```python
from build123d import *

# Parameters (mm, degrees)
F1_DEPTH = 25.4
F3_D     = 12.7
F5_D     = 12.7


with BuildPart() as f1:
    # F0 (on Front) → F1 (new body)
    with BuildSketch(Plane.XZ):
        Polygon((-34.180485, 31.123895), (-71.779169, 31.123895), (-71.779169, -31.123895), (71.779169, -31.123895), (71.779169, 31.123895), (29.286098, 31.123895), (29.286098, 4.353631), (-34.180485, 4.353631), align=None)
    extrude(amount=F1_DEPTH)

    # F3 (through all)
    with Locations(Plane.XY.offset(4.353631)):
        with Locations((0, -12.7)):
            Hole(F3_D / 2)

    # F5 (through all)
    with Locations(Plane(origin=(-71.779169, 0, 0), x_dir=(0, -1, 0), z_dir=(-1, 0, 0))):
        with Locations((12.7, 0)):
            Hole(F5_D / 2)


solid = f1.part
```
Geometry: final body of the model. Coordinates: model frame, mm. A direction names the side the tool comes from. Give positions to 0.01 mm unless a question says otherwise; leave off trailing zeros. Order: outer loops, then holes, each group sorted by start corner. A loop starts at its lowest first (then second) coordinate and runs counter-clockwise, first axis right, second up. Notation, with made-up numbers: (77.5, 89) -> (120.5, 89) arc R19 ccw to (120.5, 108) -> close; hole circle Ø11 at (-30.5, 77). An arc over 180 degrees is marked (long way). Write each question's results on one line, items separated by ' | '. Start each with the question number.
1) Draft query along Y for faces 1 (the flat face through (-1, -25.4, -6)), 2 (the flat face through (-1, 0, -6)), 3 (the cylindrical face through (-43.36, -14.08, -6.2)), 4 (the cylindrical face through (-0.07, -6.35, 2.63)). Return one class per face: pulls with the +Y half, pulls with the -Y half, needs draft (parallel to the pull), parting line crosses it, or undercut.
2) Line query: line 1 (X direction, y = -12.7, z = -9); line 2 (Y direction, x = 0, z = -21.5); line 3 (X direction, y = -2.25, z = 9.5). Output: solid intervals per line, ascending. Write a range as from..to.
3) Section D-D (x = -47). Return loops of the section in (y, z).
4) First-contact query: pin 1 (9 mm diameter, centred on x = -7.5, y = -22.5, fed in from +Z). Flat tip, straight axial feed; report the tip coordinate or a pass-through.
5) Section B-B (y = -12.7). Return loops of the section in (x, z), then the cut area to 3 significant figures.
6) Set-up query: faces 5 (the flat face through (71.779, -13, -7)), 6 (the cylindrical face through (0.07, -19.05, 2.63)), 7 (the flat face through (-2, -4, 4.354)). Return all of +Z, -Z, +X, -X, +Y, -Y with unobstructed straight access to the full face (end or side cutting, diameter ignored); none if empty.
7) Section A-A (z = 25). Return loops of the section in (x, y).
8) Section C-C (z = -14). Return loops of the section in (x, y).
Calculated:
1) face 1: pulls with the -Y half | face 2: pulls with the +Y half | face 3: undercut | face 4: undercut
2) line 1: -71.78..-6.35, 6.35..71.78 | line 2: -25.4..-19.05, -6.35..0 | line 3: -71.78..-34.18, 29.29..71.78
3) outline: (-25.4, -31.12) -> (0, -31.12) -> (0, 31.12) -> (-25.4, 31.12) -> close; hole circle Ø12.7 at (-12.7, 0)
4) pin 1: z = 4.35
5) outline: (-71.78, -31.12) -> (-6.35, -31.12) -> (-6.35, -6.35) -> (-71.78, -6.35) -> close; (-71.78, 6.35) -> (-34.18, 6.35) -> (-34.18, 31.12) -> (-71.78, 31.12) -> close; (6.35, -31.12) -> (71.78, -31.12) -> (71.78, -6.35) -> (6.35, -6.35) -> close; (29.29, 6.35) -> (71.78, 6.35) -> (71.78, 31.12) -> (29.29, 31.12) -> close | area: 5,230 mm2
6) face 5: +Z, -Z, +X, +Y, -Y | face 6: +Z, -Z | face 7: +Z, +Y, -Y
7) outline: (-71.78, -25.4) -> (-34.18, -25.4) -> (-34.18, 0) -> (-71.78, 0) -> close; (29.29, -25.4) -> (71.78, -25.4) -> (71.78, 0) -> (29.29, 0) -> close
8) outline: (-71.78, -25.4) -> (71.78, -25.4) -> (71.78, 0) -> (-71.78, 0) -> close; hole circle Ø12.7 at (0, -12.7)
